Input: part model. Units: mm. Frame: model coordinates. A direction names the side the tool comes from. Coordinates: 2 decimals unless noted, no trailing zeros. Loops run counter-clockwise (first coordinate to the right, second up) from the corner with the lowest first, then second, coordinate; pieces in that order, holes last. Notation, with made-up numbers: M 89.5,-9.75 L 97.5,-9.75 A20 cw 97.5,27.25 Z; hole C -22,88.25 d6. An arc over 180 degrees is marked long. Use a Markdown table: item, result. Add a question column.
1. Set-up query: faces 4 (the flat face through (-338, -143.657, 526)), 5 (the flat face through (156, 1, -86.489)), 6 (the flat face through (332.205, -129, 397)). Return all of +Z, -Z, +X, -X, +Y, -Y with unobstructed straight access to the full face (end or side cutting, diameter ignored); none if empty.
2. Section B-B on z = -24.5. Output: boundary loops of the cut face in (x, y).
3. Section D-D on y = 53.5. Output: boundary loops of the cut face in (x, z), then the cut area to 3 significant figures.
4. Section C-C on y = -93. Output: boundary loops of the cut face in (x, z).
5. Section A-A on x = 279.5. Output: boundary loops of the cut face in (y, z).
6. Pin query (flat end, axial travel): pin 1 (4 mm diameter, centred on x = 56.5, y = -260.5, fed in from +Z); pin 2 (4 mm diameter, centred on x = -352.5, z = 573, fed in from -Y); pin 3 (3 mm diameter, centred on x = -335.5, z = 287.5, fed in from -Y). Return the tip coordinate at first contact, or that it passes through.
7. Line query: L1, parallel to Z at x = -25, y = -39; L2, parallel to X at y = 267, z = 0.5; L3, parallel to Z at x = -83, y = -272. Output: solid intervals per line, ascending. Write a range as [from, to].
8. Draft query along Y for faces 1 (the flat face through (-87.243, 103, 361)), 2 (the flat face through (76, -343.657, -108)), 3 (the flat face through (-582.104, -223, 482)). Return one class per face: +Y half, -Y half, draft (parallel to the pull), parting line (faces both ways), or undercut.
```python
from build123d import *

# Parameters (mm, degrees)
SKETCH_1_W          = 165
SKETCH_1_H          = 70
EXTRUDE_1_DEPTH     = 116
SKETCH_2_W          = 100
SKETCH_2_H          = 40
CUT_EXTRUDE_1_DEPTH = 170.680327977
CUT_EXTRUDE_2_DEPTH = 70
SKETCH_4_W          = 49.486084661
SKETCH_4_H          = 20
CUT_EXTRUDE_3_DEPTH = 40
SKETCH_5_W          = 90
SKETCH_5_H          = 20
CUT_EXTRUDE_4_DEPTH = 20
SKETCH_6_R          = 12.5
EXTRUDE_2_DEPTH     = 20
SKETCH_7_W          = 100
SKETCH_7_H          = 15
CUT_EXTRUDE_5_DEPTH = 20
SKETCH_8_W          = 30
SKETCH_8_H          = 20
EXTRUDE_3_DEPTH     = 30
CUT_EXTRUDE_6_DEPTH = 30
SKETCH_10_R         = 12.5
EXTRUDE_5_DEPTH     = 5
SKETCH_11_W         = 90
SKETCH_11_H         = 10
CUT_EXTRUDE_7_DEPTH = 170.680327977
SKETCH_12_W         = 19.793287236
SKETCH_12_H         = 19.804361638
EXTRUDE_6_DEPTH     = 15
SKETCH_13_R         = 11.356941905
SKETCH_13_R_2       = 5.84992953
EXTRUDE_7_DEPTH     = 5
SKETCH_14_R         = 3.636100405
EXTRUDE_8_DEPTH     = 5
SCALE_1_SCALE       = 10


with BuildPart() as part:
    # ｽｹｯﾁ1 → ﾎﾞｽ - 押し出し1 (new body)
    with BuildSketch(Plane.XY):
        with Locations((19.653872675, 23.252863688)):
            Rectangle(SKETCH_1_W, SKETCH_1_H)
    extrude(amount=EXTRUDE_1_DEPTH)

    # ｽｹｯﾁ2 → ｶｯﾄ - 押し出し1 (cut, through all)
    with BuildSketch(Plane(origin=(0, -11.747136312, 0), x_dir=(-1, 0, 0), z_dir=(0, -1, 0))):
        with Locations((-52.153872675, -96)):
            Rectangle(SKETCH_2_W, SKETCH_2_H)
    extrude(amount=-CUT_EXTRUDE_1_DEPTH, mode=Mode.SUBTRACT)

    # ｽｹｯﾁ3 → ｶｯﾄ - 押し出し2 (cut)
    with BuildSketch(Plane.ZY.offset(62.846127325)):
        Polygon((116, -11.747136312), (116, 8.252863688), (86, -11.747136312), align=None)
        Polygon((116, 58.252863688), (106, 58.252863688), (116, 48.252863688), align=None)
    extrude(amount=-CUT_EXTRUDE_2_DEPTH, mode=Mode.SUBTRACT)

    # ｽｹｯﾁ4 → ｶｯﾄ - 押し出し3 (cut)
    with BuildSketch(Plane.XY.offset(116)):
        with Locations((-22.589169656, -1.747136312)):
            Rectangle(SKETCH_4_W, SKETCH_4_H)
    extrude(amount=-CUT_EXTRUDE_3_DEPTH, mode=Mode.SUBTRACT)

    # ｽｹｯﾁ5 → ｶｯﾄ - 押し出し4 (cut)
    with BuildSketch(Plane(origin=(0, -11.747136312, 0), x_dir=(-1, 0, 0), z_dir=(0, -1, 0))):
        with Locations((-19.653872675, -10)):
            Rectangle(SKETCH_5_W, SKETCH_5_H)
    extrude(amount=-CUT_EXTRUDE_4_DEPTH, mode=Mode.SUBTRACT)

    # ｽｹｯﾁ6 → ﾎﾞｽ - 押し出し2 (add)
    with BuildSketch(Plane(origin=(2.153872675, 0, 0), x_dir=(0, 0, -1), z_dir=(1, 0, 0))):
        with Locations(Location((-96, 33.252863688, 0), (0, 0, 180))):
            Circle(SKETCH_6_R)
    extrude(amount=EXTRUDE_2_DEPTH)

    # ｽｹｯﾁ7 → ｶｯﾄ - 押し出し5 (cut)
    with BuildSketch(Plane.XY.offset(76)):
        with Locations((52.153872675, 33.252863688)):
            Rectangle(SKETCH_7_W, SKETCH_7_H)
    extrude(amount=-CUT_EXTRUDE_5_DEPTH, mode=Mode.SUBTRACT)

    # ｽｹｯﾁ8 → ﾎﾞｽ - 押し出し3 (add)
    with BuildSketch(Plane.XY.offset(76)):
        with Locations((82.153872675, 33.252863688)):
            Rectangle(SKETCH_8_W, SKETCH_8_H)
    extrude(amount=EXTRUDE_3_DEPTH)

    # ｽｹｯﾁ9 → ｶｯﾄ - 押し出し6 (cut)
    with BuildSketch(Plane(origin=(97.153872675, 0, 0), x_dir=(0, 0, -1), z_dir=(1, 0, 0))):
        with BuildLine():
            ThreePointArc((-106, 33.252863688), (-103.071067812, 40.3239315), (-96, 43.252863688))
            Line((-96, 43.252863688), (-106, 43.252863688))
            Line((-106, 43.252863688), (-106, 33.252863688))
        make_face()
        with BuildLine():
            ThreePointArc((-96, 23.252863688), (-103.071067812, 26.181795877), (-106, 33.252863688))
            Line((-106, 33.252863688), (-106, 23.252863688))
            Line((-106, 23.252863688), (-96, 23.252863688))
        make_face()
    extrude(amount=-CUT_EXTRUDE_6_DEPTH, mode=Mode.SUBTRACT)

    # ｽｹｯﾁ10 → ﾎﾞｽ - 押し出し5 (add)
    with BuildSketch(Plane(origin=(97.153872675, 0, 0), x_dir=(0, 0, -1), z_dir=(1, 0, 0))):
        with Locations(Location((-96, 33.252863688, 0), (0, 0, 180))):
            Circle(SKETCH_10_R)
    extrude(amount=EXTRUDE_5_DEPTH)

    # ｽｹｯﾁ11 → ｶｯﾄ - 押し出し7 (cut, through all)
    with BuildSketch(Plane.XZ.offset(11.747136312)):
        with Locations((27.153872675, 40)):
            Rectangle(SKETCH_11_W, SKETCH_11_H)
    extrude(amount=-CUT_EXTRUDE_7_DEPTH, mode=Mode.SUBTRACT)

    # ｽｹｯﾁ12 → ﾎﾞｽ - 押し出し6 (add)
    with BuildSketch(Plane.XY.offset(76)):
        with Locations((53.995302242, 9.902180819)):
            Rectangle(SKETCH_12_W, SKETCH_12_H)
    extrude(amount=EXTRUDE_6_DEPTH)

    # ｽｹｯﾁ13 → ﾎﾞｽ - 押し出し7 (add)
    with BuildSketch(Plane(origin=(0, -11.747136312, 0), x_dir=(-1, 0, 0), z_dir=(0, -1, 0))):
        with Locations(Location((-20.471789783, -64.844641849, 0), (0, 0, 280.811331396))):
            Circle(SKETCH_13_R)
        with Locations(Location((-48.379056958, -62.343196008, 0), (0, 0, 270))):
            Circle(SKETCH_13_R_2)
    extrude(amount=EXTRUDE_7_DEPTH)

    # ｽｹｯﾁ14 → ﾎﾞｽ - 押し出し8 (add)
    with BuildSketch(Plane(origin=(63.89194586, 0, 0), x_dir=(0, 0, -1), z_dir=(1, 0, 0))):
        with Locations(Location((-86.03727841, 6.236286701, 0), (0, 0, 180))):
            Circle(SKETCH_14_R)
    extrude(amount=EXTRUDE_8_DEPTH)


with BuildPart() as part_1:
    # ｽｹｰﾙ1: scaled about (12.08683356, 25.131751334, 48.498774543)
    add(part.part.scale(SCALE_1_SCALE).moved(Location((-108.78150204, -226.185762006, -436.488970887))))


solid = part_1.part
```
Answers below:
| question | item | result |
|---|---|---|
| 1 | face 4 | +Z, -Y |
| 1 | face 5 | +Y, -Y |
| 1 | face 6 | +Z, +Y, -Y |
| 2 | outline | M -737.24,-343.66 L -287.24,-343.66 L -287.24,356.34 L -737.24,356.34 Z; M 612.76,-343.66 L 912.76,-343.66 L 912.76,356.34 L 612.76,356.34 Z |
| 3 | outline | M -737.24,-436.49 L 912.76,-436.49 L 912.76,123.51 L -87.24,123.51 L -87.24,410.23 L 112.76,410.23 L 112.76,636.79 L -87.24,636.79 L -87.24,723.51 L -737.24,723.51 Z; M 562.76,323.51 L 862.76,323.51 L 862.76,410.23 L 912.76,410.23 L 912.76,636.79 L 862.76,636.79 L 862.76,608.41 L 562.76,608.41 Z; hole M -287.24,-86.49 L 612.76,-86.49 L 612.76,13.51 L -287.24,13.51 Z |
| 3 | area | 1,370,000 mm² |
| 4 | outline | M -737.24,-436.49 L 912.76,-436.49 L 912.76,323.51 L 530.14,323.51 L 530.14,473.51 L 332.21,473.51 L 332.21,323.51 L -87.24,323.51 L -87.24,723.51 L -737.24,723.51 Z; hole M -287.24,-86.49 L 612.76,-86.49 L 612.76,13.51 L -287.24,13.51 Z |
| 5 | outline | M -343.66,-236.49 L -143.66,-236.49 L -143.66,-436.49 L 356.34,-436.49 L 356.34,-86.49 L -343.66,-86.49 Z; M -343.66,13.51 L 356.34,13.51 L 356.34,323.51 L 181.34,323.51 L 181.34,123.51 L 31.34,123.51 L 31.34,323.51 L -343.66,323.51 Z |
| 6 | pin 1 | stops at z = 323.51 |
| 6 | pin 2 | stops at y = -143.66 |
| 6 | pin 3 | stops at y = -343.66 |
| 7 | L1 | z = [-436.49, -86.49], [13.51, 323.51] |
| 7 | L2 | x = [-737.24, -287.24], [612.76, 912.76] |
| 7 | L3 | z = [-236.49, -86.49], [13.51, 323.51] |
| 8 | face 1 | undercut |
| 8 | face 2 | -Y half |
| 8 | face 3 | draft |
